Can you work these out from the model? Positions are in its coordinate system, mm. Face numbers are marked on the shaded views. A direction names the side the tool comes from. Coordinates: 2 decimals unless noted, no trailing zeros. Loops run counter-clockwise (first coordinate to the right, second up) from the corner with the lowest first, then second, coordinate; pieces in that order, holes last.
```python
from build123d import *

# Parameters (mm, degrees)
F1_DEPTH = 25
F2_DEPTH = 10


with BuildPart() as f1:
    # F0 (on Front) → F1 (new body)
    with BuildSketch(Plane.XZ):
        with BuildLine():
            ThreePointArc((15, 150), (0, 165), (-15, 150))
            Line((-15, 150), (15, 150))
        make_face()
        with BuildLine():
            Line((15, 150), (-15, 150))
            ThreePointArc((-15, 150), (0, 135), (15, 150))
        make_face()
    extrude(amount=F1_DEPTH)

    # F0 (on Front) → F2 (join)
    with BuildSketch(Plane.XZ):
        with BuildLine():
            ThreePointArc((15, 150), (0, 165), (-15, 150))
            Line((-15, 150), (15, 150))
        make_face()
        with BuildLine():
            ThreePointArc((15, 150), (0, 135), (-15, 150))
            Line((-15, 150), (-15, -50))
            Line((-15, -50), (15, -50))
            Line((15, -50), (15, 150))
        make_face()
    extrude(amount=F2_DEPTH)


solid = f1.part
```
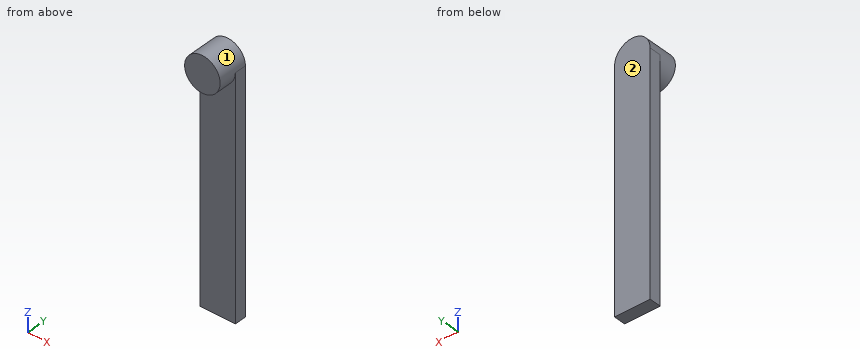
(1) I'm going to push flat-ended pins straight in: pin 1 (3 mm diameter, centred on x = 8, y = -10.5, fed in from +Z); pin 2 (3 mm diameter, centred on x = 10.5, y = -7.5, fed in from +Z); pin 3 (4 mm diameter, centred on x = -11.5, y = -22, fed in from -Z). Where does each tip first touch, or does it pass through?
Check values:
pin 1: stops at z = 163.52
pin 2: stops at z = 162
pin 3: stops at z = 138.39
(2) If I drill on probe 1 along Y at (x, z) = (-8.5, 103.5); probe 2 along X at (y, z) = (-16, 141); probe 3 along Z at (x, y) = (0.5, -23), over which ranges is the centre line in solid material (lowest first)?
Check values:
probe 1: y = -10 to 0
probe 2: x = -12 to 12
probe 3: z = 135.01 to 164.99
(3) I want a section at C-C on y = -15.5. Write out the boundary of the cut face in (x, z).
Check values:
outline: circle Ø30 at (0, 150)
(4) I want a section at D-D on z = 79. Write out the boundary of the cut face in (x, y).
Check values:
outline: (-15, -10) - (15, -10) - (15, 0) - (-15, 0) - close
(5) Which directions (+Z, -Z, +X, -X, +Y, -Y) give clear straight access to the entire face, cutting with the end or side of a thin tool? Please do the marked faces 1 and 2.
Check values:
face 1: -Y
face 2: +Z, -Z, +X, -X, +Y
(6) I want a section at B-B on z = 142. Write out the boundary of the cut face in (x, y), then the cut area to 3 significant figures.
Check values:
outline: (-15, -10) - (-12.69, -10) - (-12.69, -25) - (12.69, -25) - (12.69, -10) - (15, -10) - (15, 0) - (-15, 0) - close
area: 681 mm2
(7) I want a section at A-A on x = 0. Write out the boundary of the cut face in (y, z).
Check values:
outline: (-25, 135) - (-10, 135) - (-10, -50) - (0, -50) - (0, 165) - (-25, 165) - close
